Work out the finished part from the listing and answer in its coordinate system (mm). A direction names the side the tool comes from. Coordinates: 2 decimals unless noted, no trailing zeros. Write each loop counter-clockwise with the first axis right and the second up, starting at its lowest first coordinate (ties: lowest second). Pieces come first, ordered by that corner, then holes. Notation, with made-up numbers: (-28.75, 33.25) - (-9.75, 33.25) arc R15 cw to (-9.75, 55.25) - close; hole circle Ø11 at (-24.75, 1.25). An arc over 180 degrees is marked (long way). Use a Markdown table: item, result. Add a question column.
(1) The part is cut by section B-B, the plane y = 229.5. Give the vertices of the cut face in (x, z), then the cut area to 3 significant figures.
(2) A tool of negligible diameter and unlimited length cuts with its end or side. For faces 1 (the face through (87, 129, 0)), 2 (the face through (0, 125.8, 0.3)), from which of +Z, -Z, +X, -X, +Y, -Y can it reach the whole face along a straight path? Write none if from no direction.
(3) Given pin 1 Ø2.5 at (x, y) = (153.862, 178.82) entering from +Z; pin 2 Ø5 at (x, y) = (153.862, 198.82) entering from -Z; pin 3 Ø1.5 at (x, z) = (46.5, -4.5) entering from +Y, each flat-ended and moving along its own axis, determine where each tip first touches the part or whether it passes through.
(4) The part is cut by section A-A, the plane x = 123. Give the vertices of the cut face in (y, z).
(5) The part is cut by section C-C, the plane z = -8.25. Give the vertices of the cut face in (x, y), then the cut area to 3 significant figures.
(6) Find the intervals of material crossed by line 1 (X direction, y = 188.82, z = 0.3); line 2 (X direction, y = 168.36, z = 0.15); line 3 (Y direction, x = 35, z = -8), in increasing order. Write a range as from..to.
Autodesk Inventor part; units mm, degrees
ref_plane "YZ Plane" through (0, 0, 0) normal (1, 0, 0) x (0, 1, 0)
ref_plane "XZ Plane" through (0, 0, 0) normal (0, 1, 0) x (-1, 0, 0)
ref_plane "XY Plane" through (0, 0, 0) normal (0, 0, 1) x (1, 0, 0)
sketch "Sketch1" plane through (0, 0, 0) normal (0, 0, 1) x (1, 0, 0)
  line L0 (0, 0) -> (181.174, 0)
  line L1 (181.174, 0) -> (181.174, 253.26)
  line L2 (181.174, 253.26) -> (0, 253.26)
  line L3 (0, 253.26) -> (0, 0)
  dimension "d0" = 181.174
  dimension "d1" = 253.26
extrude "Plate1" add sketch "Sketch1" along normal blind 0.5
sketch "Sketch3" plane through (0, 0, 0.5) normal (0, 0, 1) x (1, 0, 0)
  line L0 (181.174, 253.26) -> (181.174, 0)
  line L1 (181.174, 253.26) -> (181.174, 168.36) construction
  line L2 (181.174, 168.36) -> (169.327, 168.36) construction
  line L3 (169.327, 168.36) -> (11.847, 168.36) construction
  line L4 (169.327, 168.36) -> (169.327, 13.48) construction
  circle A0 centre (169.327, 13.48) radius 1.5
  circle A1 centre (169.327, 168.36) radius 1.5
  circle A2 centre (11.847, 168.36) radius 1.5
  point P0 (181.174, 0.5)
  point P1 (0, 0)
  dimension "d13" = 84.9
  dimension "d14" = 11.847
  dimension "d15" = 157.48
  dimension "d16" = 154.88
  dimension "d17" = 3
  dimension "d18" = 3
  dimension "d19" = 3
extrude "Extrusion1" cut sketch "Sketch3" against normal blind 10
sketch "Sketch5" plane through (0, 0, 0.5) normal (0, 0, 1) x (1, 0, 0)
  circle A0 centre (11.847, 168.36) radius 1.5
  line L0 (11.847, 168.36) -> (11.847, 35.808) construction
  line L1 (11.847, 168.36) -> (144.399, 168.36) construction
  line L2 (11.847, 35.808) -> (11.847, 36.34) construction
  circle A1 centre (11.847, 36.34) radius 1.5
  point P0 (0, 0)
  dimension "d28" = 90
  dimension "d32" = 0.532
  dimension "d33" = 3
extrude "Extrusion4" cut sketch "Sketch5" against normal blind 10 contours A1
sketch "Sketch7" plane through (0, 0, 0) normal (0, -1, 0) x (1, 0, 0)
  line L0 (181.174, 0) -> (0, 0)
  line L1 (0, 0) -> (0, -10.5)
  line L2 (0, -10.5) -> (181.174, -10.5)
  line L3 (181.174, -10.5) -> (181.174, 0)
edge flange "Flange2" height 11 angle 90 thickness 0.5 bend radius 0.5 thickness toward (0, -1, 0) relief tear relief width 0.5 relief depth 0.25 edges at (90.587, 0, 0) wall of the first edge with corners at (181.174, 0, 0) (0, 0, 0) (0, 0, -10.5) (181.174, 0, -10.5)
bend "Bend2"
corner "Corner2"
sketch "Sketch8" plane through (0, 0, 0.5) normal (0, 0, 1) x (1, 0, 0)
  line L0 (181.174, 253.26) -> (0, 253.26)
  line L1 (181.174, 253.26) -> (177.174, 253.26)
  line L2 (177.174, 253.26) -> (177.174, -19.1311)
  line L3 (177.174, -19.1311) -> (181.174, -19.1311)
  line L4 (181.174, -19.1311) -> (181.174, 253.26)
  point P0 (0, 0)
  dimension "d46" = 4
extrude "Extrusion5" cut sketch "Sketch8" against normal through all
sketch "Sketch9" plane through (0, 0, 0.5) normal (0, 0, 1) x (1, 0, 0)
  line L0 (177.174, 253.26) -> (177.174, 198.82) construction
  line L1 (177.174, 253.26) -> (177.174, 0.5) construction
  line L2 (177.174, 198.82) -> (153.862, 198.82) construction
  circle A0 centre (153.862, 198.82) radius 1.5
  line L3 (153.862, 198.82) -> (153.862, 188.82) construction
  line L4 (153.862, 188.82) -> (153.862, 178.82) construction
  circle A1 centre (153.862, 188.82) radius 1.5
  circle A2 centre (153.862, 178.82) radius 1.5
  line L5 (153.862, 198.82) -> (38.862, 198.82) construction
  circle A3 centre (38.862, 198.82) radius 1.5
  circle A4 centre (38.862, 188.82) radius 1.5
  circle A5 centre (38.862, 178.82) radius 1.5
  point P0 (0, 0)
  dimension "d49" = 54.44
  dimension "d50" = 23.312
  dimension "d55" = 3
  dimension "d58" = 10
  dimension "d59" = 10
  dimension "d60" = 3
  dimension "d61" = 3
  dimension "d62" = 115
  dimension "d63" = 3
  dimension "d64" = 3
  dimension "d65" = 3
extrude "Extrusion7" cut sketch "Sketch9" against normal blind 10
sketch "Sketch10" plane through (0, 0, 0.5) normal (0, 0, 1) x (1, 0, 0)
  circle A0 centre (153.862, 198.82) radius 1.5
  circle A1 centre (38.862, 198.82) radius 1.5
  line L0 (38.862, 198.82) -> (48.862, 198.82) construction
  line L1 (153.862, 198.82) -> (143.862, 198.82) construction
  line L2 (48.862, 198.82) -> (143.862, 198.82)
  line L3 (143.862, 198.82) -> (143.862, 178.82)
  line L4 (143.862, 178.82) -> (48.862, 178.82)
  line L5 (48.862, 178.82) -> (48.862, 198.82)
  point P0 (0, 0)
  dimension "d68" = 10
  dimension "d69" = 10
  dimension "d70" = 20
extrude "Extrusion8" cut sketch "Sketch10" against normal blind 10 contours L2 L3 L4 L5
equation "\"d2\" = Thickness"
equation "\"d36\" = BendReliefWidth"
equation "\"d37\" = BendReliefDepth"
equation "\"d38\" = MinimumRemnant"
equation "\"d39\" = TransitionRadius"
equation "\"d42\" = BendRadius"
equation "\"d43\" = CornerReliefSize"
equation "\"d44\" = GapSize"
equation "\"d45\" = JacobiRadiusSize"
equation "\"BendRadius\" = Thickness"
equation "\"BendReliefWidth\" = Thickness"
equation "\"BendReliefDepth\" = 0.5 * Thickness"
equation "\"CornerReliefSize\" = 4 * Thickness"
equation "\"MinimumRemnant\" = 2 * Thickness"
equation "\"TransitionRadius\" = BendRadius"
equation "\"JacobiRadiusSize\" = BendRadius"
equation "\"GapSize\" = Thickness"
properties part number "dads trunk"
Model answer:
| question | item | result |
|---|---|---|
| 1 | outline | (0, 0) - (177.17, 0) - (177.17, 0.5) - (0, 0.5) - close |
| 1 | area | 88.6 mm^2 |
| 2 | face 1 | -Z, +X, -X, +Y |
| 2 | face 2 | +Z, -Z, -X, +Y, -Y |
| 3 | pin 1 | through |
| 3 | pin 2 | z = 0 |
| 3 | pin 3 | y = 0 |
| 4 | outline | (-0.5, -10.5) - (0, -10.5) - (0, -0.5) arc R0.5 cw to (0.5, 0) - (178.82, 0) - (178.82, 0.5) - (0.5, 0.5) arc R1 ccw to (-0.5, -0.5) - close; (198.82, 0) - (253.26, 0) - (253.26, 0.5) - (198.82, 0.5) - close |
| 5 | outline | (0, -0.5) - (177.17, -0.5) - (177.17, 0) - (0, 0) - close |
| 5 | area | 88.6 mm^2 |
| 6 | line 1 | 0..37.36, 40.36..48.86, 143.86..152.36, 155.36..177.17 |
| 6 | line 2 | 0..10.35, 13.35..167.83, 170.83..177.17 |
| 6 | line 3 | -0.5..0 |
